Input: part model. Units: mm. Frame: model coordinates. Round coordinates to 2 decimals unless told otherwise and drop trailing zeros. Loops run counter-clockwise (first coordinate to the right, second up) from the corner with the lowest first, then second, coordinate; pieces in that order, holes last. Notation, with made-up numbers: M -37.75,70 L -17.75,70 A32 cw -17.75,97 Z; hole C 81,-40 d2. An arc over 180 degrees is marked long. Put each result on its own line as item: value. Start each with the question number.
1) Draft query along X for faces 1 (the face through (-1.86, 7.64, 14.18)), 2 (the face through (-5.8, 10, 16.4)), 3 (the face through (-2.22, 5.563, 16.905)), 4 (the face through (-14.985, 18.704, 0.66)). Return one class per face: +X half, -X half, draft (parallel to the pull), parting line (faces both ways), or undercut.
2) Pin query (flat end, axial travel): pin 1 (3 mm diameter, centred on x = -17, z = -17.5, fed in from -Y); pin 2 (10 mm diameter, centred on x = 14.5, y = 11.5, fed in from -Z); pin 3 (8 mm diameter, centred on x = 17, z = 12, fed in from -Y); pin 4 (17 mm diameter, centred on x = 0, z = 0, fed in from -Y). Return the tip coordinate at first contact, or that it passes through.
3) Section A-A on x = 0. Output: boundary loops of the cut face in (y, z).
4) Section B-B on z = 0. Output: boundary loops of the cut face in (x, y).
5) Line query: probe 1 along Z at (x, y) = (0, 8.5); probe 2 along Y at (x, z) = (18.5, -5.5); probe 3 along Z at (x, y) = (-15.5, 14.25). Output: solid intervals per line, ascending.
from build123d import *

# Parameters (mm, degrees)
CHAMFER1_SIZE = 3
CHAMFER2_SIZE = 1


with BuildPart() as part:
    # Sketch1 → Revolve1 (revolve)
    with BuildSketch(Plane.XY):
        Polygon((14.3, 0), (17.05, 0), (17.05, 10), (23.05, 10), (23.05, 22), (15, 22), (15, 15.5), (14.3, 15.5), align=None)
    revolve(axis=Axis((0, 23.1, 0), (0, -1, 0)))

    # Chamfer1
    chamfer1_edges = [part.edges().sort_by_distance(p)[0] for p in [
        (-23.05, 22, 0),
        (-23.05, 10, 0),
    ]]
    chamfer(chamfer1_edges, length=CHAMFER1_SIZE)

    # Chamfer2
    chamfer2_edges = [part.edges().sort_by_distance(p)[0] for p in [
        (-17.05, 0, 0),
    ]]
    chamfer(chamfer2_edges, length=CHAMFER2_SIZE)


solid = part.part
Geometry results:
1. face 1: undercut
1. face 2: draft
1. face 3: parting line
1. face 4: undercut
2. pin 1: stops at y = 12.85
2. pin 2: stops at z = -20.9
2. pin 3: stops at y = 0.76
2. pin 4: passes through
3. outline: M 0,-16.05 L 1,-17.05 L 10,-17.05 L 10,-20.05 L 13,-23.05 L 19,-23.05 L 22,-20.05 L 22,-15 L 15.5,-15 L 15.5,-14.3 L 0,-14.3 Z; M 0,14.3 L 15.5,14.3 L 15.5,15 L 22,15 L 22,20.05 L 19,23.05 L 13,23.05 L 10,20.05 L 10,17.05 L 1,17.05 L 0,16.05 Z
4. outline: M -23.05,13 L -20.05,10 L -17.05,10 L -17.05,1 L -16.05,0 L -14.3,0 L -14.3,15.5 L -15,15.5 L -15,22 L -20.05,22 L -23.05,19 Z; M 14.3,0 L 16.05,0 L 17.05,1 L 17.05,10 L 20.05,10 L 23.05,13 L 23.05,19 L 20.05,22 L 15,22 L 15,15.5 L 14.3,15.5 Z
5. probe 1: z = -17.05 to -14.3, 14.3 to 17.05
5. probe 2: y = 10 to 22
5. probe 3: z = -17.06 to 17.06
